```python
from build123d import *

# Parameters (mm, degrees)
F1_DEPTH = 6
F2_R     = 1.65
F3_DEPTH = 25
F4_R     = 2


with BuildPart() as f1:
    # F0 (on Top) → F1 (new body)
    with BuildSketch(Plane.XY):
        with BuildLine():
            Line((-0.5, 7), (-3.5, 7))
            Line((-3.5, 7), (-3.5, -3))
            Line((-3.5, -3), (3.5, -3))
            Line((3.5, -3), (3.5, 7))
            Line((3.5, 7), (0.5, 7))
            Line((0.5, 7), (0.5, 1.361066))
            ThreePointArc((0.5, 1.361066), (1.189012, 0.82991), (1.45, 0))
            ThreePointArc((1.45, 0), (-0.82991, -1.189012), (-0.5, 1.361066))
            Line((-0.5, 1.361066), (-0.5, 7))
        make_face()
    extrude(amount=F1_DEPTH)

    # F2 (on face) → F3 (cut)
    with BuildSketch(Plane.YZ.offset(3.5)):
        with Locations((4, 3)):
            Circle(F2_R)
    extrude(amount=-F3_DEPTH, mode=Mode.SUBTRACT)

    # F4
    f4_edges = [f1.edges().sort_by_distance(p)[0] for p in [
        (3.5, -3, 3),
        (-3.5, -3, 3),
    ]]
    fillet(f4_edges, radius=F4_R)


solid = f1.part
```
Can you work these out from the model? Positions are in its coordinate system, mm. A direction names the side the tool comes from. Give positions to 0.01 mm unless a question says otherwise; leave off trailing zeros. Loops run counter-clockwise (first coordinate to the right, second up) from the corner with the lowest first, then second, coordinate; pieces in that order, holes last. Notation, with made-up numbers: M 71,79.5 L 129,79.5 A36 cw 129,116.5 Z; hole C 48.25,43.5 d1. An arc over 180 degrees is marked long. Use CSV: the item, a comma, the result in double quotes. Start each with the question number.
1. Imagine slicing it at D-D, the plane z = 0.4. Write out the boundary of the cut face in (x, y).
2. For P1, Ø1.5, axis at y = -1.5, z = 1, coming from the +X side, with a flat end and sliding along its axis, tell me the tip position at first contact or that it passes through.
3. If we mould it in two halves opening along Z, with no side actions, what happens to faces 3 (the face through (-2.93, -2.4, 3.04)), 4 (the face through (1, 2, 0)), 5 (the face through (-1.979, 2.784, 4.115)), 6 (the face through (1, 2, 6))? For each: released by +Z, released by -Z, zero draft, split by the parting line, or undercut.
4. If I drill on L1, parallel to X at y = 2, z = 3.75; L2, parallel to Z at x = 2.1, y = 4; L3, parallel to X at y = -0.5, z = 2.3, over which ranges is the centre line in solid material (lowest first)?
5. On a 3-axis mill with a long thin cutter (end or side, diameter ignored), from which of +Z, -Z, +X, -X, +Y, -Y can I reach the whole of each face in a straight line? I mean faces 1 (the face through (3.5, 2, 3)), 2 (the face through (0.5, 5.5, 1.6)). Say none if no direction works.
6. Imagine slicing it at C-C, the plane y = 4. Write out the boundary of the cut face in (x, z).
7. Imagine slicing it at B-B, the plane z = 3. Write out the boundary of the cut face in (x, y), plus the area to 3 significant figures.
8. Imagine slicing it at A-A, the plane y = 1. Write out the boundary of the cut face in (x, z), plus the area to 3 significant figures.
Response values:
1,outline,"M -3.5,-1 A2 ccw -1.5,-3 L 1.5,-3 A2 ccw 3.5,-1 L 3.5,7 L 0.5,7 L 0.5,1.36 A1.45 cw long -0.5,1.36 L -0.5,7 L -3.5,7 Z"
2,P1,"x = 3.5"
3,face 3,"zero draft"
3,face 4,"released by -Z"
3,face 5,"undercut"
3,face 6,"released by +Z"
4,L1,"-3.5 to -0.5, 0.5 to 3.5"
4,L2,"0 to 1.35, 4.65 to 6"
4,L3,"-3.5 to -1.36, 1.36 to 3.5"
5,face 1,"+Z, -Z, +X, +Y, -Y"
5,face 2,"+Z, -Z, +Y"
6,outline,"M -3.5,0 L -0.5,0 L -0.5,1.35 L -3.5,1.35 Z; M -3.5,4.65 L -0.5,4.65 L -0.5,6 L -3.5,6 Z; M 0.5,0 L 3.5,0 L 3.5,1.35 L 0.5,1.35 Z; M 0.5,4.65 L 3.5,4.65 L 3.5,6 L 0.5,6 Z"
7,outline,"M -3.5,-1 A2 ccw -1.5,-3 L 1.5,-3 A2 ccw 3.5,-1 L 3.5,2.35 L 0.5,2.35 L 0.5,1.36 A1.45 cw long -0.5,1.36 L -0.5,2.35 L -3.5,2.35 Z; M -3.5,5.65 L -0.5,5.65 L -0.5,7 L -3.5,7 Z; M 0.5,5.65 L 3.5,5.65 L 3.5,7 L 0.5,7 Z"
7,area,"36.3 mm^2"
8,outline,"M -3.5,0 L -1.05,0 L -1.05,6 L -3.5,6 Z; M 1.05,0 L 3.5,0 L 3.5,6 L 1.05,6 Z"
8,area,"29.4 mm^2"
